Model file for the job. Use its own axes, mm. A direction names the side the tool comes from. Coordinates: 2 decimals unless noted, no trailing zeros. Order: outer loops, then holes, each group sorted by start corner. A loop starts at its lowest first (then second) coordinate and runs counter-clockwise, first axis right, second up.
from build123d import *

# Parameters (mm, degrees)
F1_DEPTH    = 21.5
F3_DEPTH    = 1
F5_DEPTH    = 1
F6_T1_DEPTH = 27.2031140795


# Not quite as in the source:
# - a fillet or chamfer that OpenCascade refuses, or shapes differently, is made with other operations: its cross-section is extruded or revolved along the edge and cut away or added


with BuildPart() as f1:
    # F0 (on Front) → F1 (new body)
    with BuildSketch(Plane.XZ):
        with BuildLine():
            Line((-3, 0), (-3, -25))
            ThreePointArc((-3, -25), (-4.4644660941, -28.5355339059), (-8, -30))
            Line((-8, -30), (-8, -30.6))
            ThreePointArc((-8, -30.6), (-4.0402020254, -28.9597979746), (-2.4, -25))
            Line((-2.4, -25), (-2.4, 0))
            ThreePointArc((-2.4, 0), (0, 2.4), (2.4, 0))
            Line((2.4, 0), (2.4, -20))
            Line((2.4, -20), (3, -20))
            Line((3, -20), (3, 0))
            ThreePointArc((3, 0), (0, 3), (-3, 0))
        make_face()
    extrude(amount=F1_DEPTH)

    # F2 (on face) → F3 (cut)
    with BuildSketch(Plane(origin=(-3, 0, 0), x_dir=(0, -1, 0), z_dir=(-1, 0, 0))):
        with BuildLine():
            Line((5.8037092493, -7.4218333804), (4.195739785, -18.3036730319))
            ThreePointArc((4.195739785, -18.3036730319), (10.75, -20.2517243137), (17.304260215, -18.3036730319))
            Line((17.304260215, -18.3036730319), (15.6962907507, -7.4218333804))
            ThreePointArc((15.6962907507, -7.4218333804), (10.75, -3.1527285914), (5.8037092493, -7.4218333804))
        make_face()
    extrude(amount=-F3_DEPTH, mode=Mode.SUBTRACT)

    # F4 (on face) → F5 (cut)
    with BuildSketch(Plane.YZ.offset(3)):
        with BuildLine():
            ThreePointArc((-13.2016747035, -12.8677467976), (-10.75, -17.5967034623), (-8.2983252965, -12.8677467976))
            ThreePointArc((-8.2983252965, -12.8677467976), (-10.75, -1.3914988898), (-13.2016747035, -12.8677467976))
        make_face()
    extrude(amount=-F5_DEPTH, mode=Mode.SUBTRACT)

    # F6: fillet of radius 2 on 1 edges, made by hand

    # F6_s2 → F6_t1 (cut)
    with BuildSketch(Plane.XZ.offset(-2.8515570398)):
        with BuildLine():
            ThreePointArc((-8, -30.6), (-7.4967757486, -30.136601148), (-6.8668213437, -29.8698979592))
            ThreePointArc((-6.8668213437, -29.8698979592), (-7.429688592, -29.9673680051), (-8, -30))
            Line((-8, -30), (-8, -30.6))
        make_face()
    extrude(amount=F6_T1_DEPTH, mode=Mode.SUBTRACT)


solid = f1.part
Q1. Drop flat-ended pins along their axis: P1, Ø1, axis at y = -11.5, z = -22, coming from the +X side; P2, Ø6, axis at y = -6.5, z = -11, coming from the -X side; P3, Ø1, axis at y = -15.5, z = -10.5, coming from the -X side; P4, Ø3.5, axis at y = -10.75, z = -14.6, coming from the +X side. Give the stop position or say it passes through.
Established:
P1: stops at x = -2.4
P2: stops at x = -3
P3: stops at x = 2.4
P4: passes through
Q2. Mould opens along Z. For faces 1 (the face through (2.4, -6, -12)), 2 (the face through (-4, -11, -28)), 3 (the face through (-2.7, -5.01, -12.79)) say: pulls with the +Z half, pulls with the -Z half, needs draft (parallel to the pull), parting line crosses it, or undercut.
Established:
face 1: needs draft
face 2: pulls with the +Z half
face 3: undercut
Q3. Which spindle directions (+Z, -Z, +X, -X, +Y, -Y) get a long thin tool onto all of the face, cutting with end or side? Do faces 4 (the face through (-2.4, -3, -13)), 5 (the face through (-2.704, -10.85, -3.154)), 6 (the face through (2.704, -10.522, -1.396)), 7 (the face through (-2.7, -10.65, -20.25)), 8 (the face through (-3, -3, -12)). Say none if no direction does.
Established:
face 4: -Z, +Y, -Y
face 5: +X, -X
face 6: +X
face 7: -X
face 8: +Z, -X, +Y, -Y
Q4. Cut at C-C, the plane x = 0. List the corners of the cut face in (y, z), plus the area to 3 significant figures.
Established:
outline: (-21.5, 2.4) - (0, 2.4) - (0, 3) - (-21.5, 3) - close
area: 12.9 mm2
Q5. Cut at A-A, the plane y = -10.75. List the corners of the cut face in (x, z), plus the area to 3 significant figures.
Established:
outline: (-8, -30.6) arc R5.6 ccw to (-2.4, -25) - (-2.4, -20.25) - (-3, -20.25) - (-3, -25) arc R5 cw to (-6.87, -29.87) arc R2 ccw to start; (-3, -3.15) - (-2.4, -3.15) - (-2.4, 0) arc R2.4 cw to (2.4, 0) - (2.4, -1.39) - (3, -1.39) - (3, 0) arc R3 ccw to (-3, 0) - close; (2.4, -20) - (3, -20) - (3, -17.6) - (2.4, -17.6) - close
area: 16.9 mm2
Q6. Cut at B-B, the plane z = -4. List the corners of the cut face in (x, y).
Established:
outline: (-3, -21.5) - (-2.4, -21.5) - (-2.4, -13.53) - (-3, -13.53) - close; (-3, -7.97) - (-2.4, -7.97) - (-2.4, 0) - (-3, 0) - close; (2.4, -21.5) - (3, -21.5) - (3, -15.7) - (2.4, -15.7) - close; (2.4, -5.8) - (3, -5.8) - (3, 0) - (2.4, 0) - close
Q7. Cut at D-D, the plane y = -6.5. List the corners of the cut face in (x, z).
Established:
outline: (-8, -30.6) arc R5.6 ccw to (-2.4, -25) - (-2.4, -19.47) - (-3, -19.47) - (-3, -25) arc R5 cw to (-6.87, -29.87) arc R2 ccw to start; (-3, -5.52) - (-2.4, -5.52) - (-2.4, 0) arc R2.4 cw to (2.4, 0) - (2.4, -3.16) - (3, -3.16) - (3, 0) arc R3 ccw to (-3, 0) - close; (2.4, -20) - (3, -20) - (3, -11.63) - (2.4, -11.63) - close
Q8. Probe line 1 (X direction, y = -5.5, z = -0.5); line 2 (X direction, y = -6.5, z = -16); line 3 (X direction, y = -12, z = 0.5). List the from-to ranges inside material, lowest first.
Established:
line 1: x = -3 to -2.4, 2.4 to 3
line 2: x = 2.4 to 3
line 3: x = -2.96 to -2.35, 2.35 to 2.96
